Autodesk Inventor part; units mm, degrees
ref_plane "YZ Plane" through (0, 0, 0) normal (1, 0, 0) x (0, 1, 0)
ref_plane "XZ Plane" through (0, 0, 0) normal (0, 1, 0) x (-1, 0, 0)
ref_plane "XY Plane" through (0, 0, 0) normal (0, 0, 1) x (1, 0, 0)
sketch "Sketch1" plane through (0, 0, 0) normal (0, 0, 1) x (1, 0, 0)
  line L0 (0, 0) -> (0, 20)
  line L1 (0, 0) -> (20, 0)
  line L2 (0, 20) -> (3, 20)
  line L3 (3, 20) -> (3, 17)
  line L4 (3, 17) -> (17, 3)
  line L5 (17, 3) -> (20, 3)
  line L6 (20, 3) -> (20, 0)
  dimension "d0" = 20
  dimension "d1" = 20
  dimension "d2" = 3
  dimension "d3" = 3
  dimension "d4" = 3
  dimension "d5" = 3
extrude "Extrusion1" add sketch "Sketch1" along normal mid plane 20
sketch "Sketch2" plane through (0, 20, 10) normal (0, 1, 0) x (1, 0, 0)
  line L0 (3, 2) -> (17, 2)
  line L1 (17, 2) -> (17, 18)
  line L2 (17, 18) -> (3, 18)
  line L3 (3, 18) -> (3, 2)
  line L4 (0, 0) -> (0, 20)
  line L5 (3, 0) -> (3, 20)
  line L6 (17, 0) -> (17, 20)
  line L7 (3, 20) -> (17, 20)
  point P0 (0, 10)
  point P1 (3, 10)
  point P2 (0, 10)
  dimension "d8" = 2
extrude "Extrusion2" cut sketch "Sketch2" against normal up to surface (17 mm away) contours L3 L2 L1 L0
sketch "Sketch3" plane through (17, 3, 10) normal (0, 1, 0) x (1, 0, 0)
  line L0 (-10, 10) -> (-3, 10) construction
  line L1 (-10, 8) -> (-3, 8)
  line L2 (-3, 12) -> (-10, 12)
  arc A0 (-10, 12) -> (-10, 8) centre (-10, 10) ccw
  arc A1 (-3, 8) -> (-3, 12) centre (-3, 10) ccw
  line L3 (-17, 0) -> (-17, 20)
  line L4 (-14, 0) -> (-14, 20)
  line L5 (3, 0) -> (3, 20)
  point P0 (-17, 10)
  point P1 (-6.5, 10)
  point P2 (-17, 10)
  point P3 (-17, 10)
  dimension "d11" = 4
  dimension "d12" = 4
  dimension "d21" = 6
extrude "Extrusion3" cut sketch "Sketch3" against normal through all
sketch "Sketch4" plane through (3, 17, 10) normal (1, 0, 0) x (0, 0, -1)
  line L0 (10, -3) -> (10, -10) construction
  line L1 (8, -3) -> (8, -10)
  line L2 (12, -10) -> (12, -3)
  arc A0 (12, -3) -> (8, -3) centre (10, -3) ccw
  arc A1 (8, -10) -> (12, -10) centre (10, -10) ccw
  line L3 (0, -17) -> (20, -17)
  line L4 (0, -14) -> (20, -14)
  line L5 (0, 3) -> (20, 3)
  point P0 (10, -17)
  point P1 (10, -6.5)
  point P2 (10, -17)
  dimension "d16" = 4
  dimension "d17" = 4
  dimension "d18" = 6
extrude "Extrusion4" cut sketch "Sketch4" against normal through all
equation "\"d1\" = d0"
equation "\"d5\" = d2"
properties part number "GUSSET 2020"
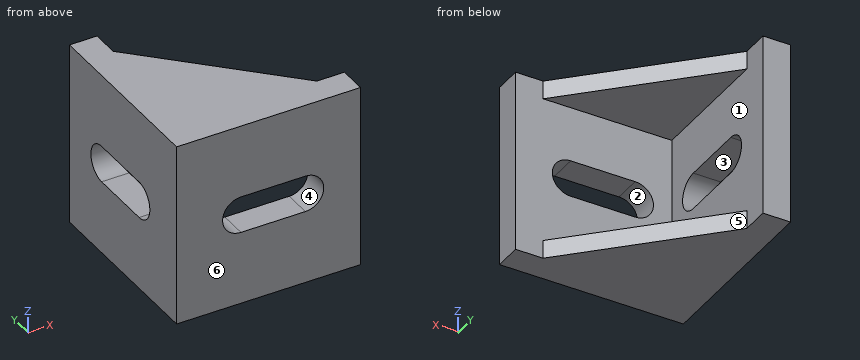
Source: CAD feature listing. Evaluate the final solid. Frame: model axes, mm. Face numbers are marked on the shaded views. A direction names the side the tool comes from. Give positions to 0.01 mm unless a question says otherwise; leave off trailing zeros. Write each loop counter-clockwise with the first axis right and the second up, starting at its lowest first coordinate (ties: lowest second). Pieces come first, ordered by that corner, then holes. Notation, with made-up numbers: (63, -37) - (116, -37) arc R22 ccw to (116, -26) - close; hole circle Ø7 at (33, -21). An arc over 180 degrees is marked (long way). One line per item, written item: value. Start each with the question number.
Q1. Section query B-B, the plane z = 0. Return the cut outline in (x, y).
Q2. Section query A-A, the plane x = 7.5. Return the cut outline in (y, z).
Q3. First-contact query: pin 1 Ø2 at (y, z) = (6.5, 7.5) entering from -X; pin 2 Ø2 at (y, z) = (14.5, 6.5) entering from +X; pin 3 Ø8.5 at (x, z) = (7.5, 0) entering from +Y. Flat tips, straight axial feed; report the tip coordinate or a pass-through.
Q4. Section query C-C, the plane x = 2.25. Return the cut outline in (y, z).
Q5. Draft query along X for the marked faces 4, 5 and 6. Return one class per face: +X half, -X half, draft (parallel to the pull), parting line (faces both ways), or undercut.
Q6. Material intervals for probe 1 along Z at (x, y) = (14.25, 5.5); probe 2 along Y at (x, z) = (5, -5.75); probe 3 along Z at (x, y) = (2, 10.5), sorted ascending. Write a range as from..to.
Q7. Set-up query: the marked faces 1, 2 and 3. Return all of +Z, -Z, +X, -X, +Y, -Y with unobstructed straight access to the full face (end or side cutting, diameter ignored); none if empty.
Q8. Section query D-D, the plane z = 8.75. Return the cut outline in (x, y), then the cut area to 3 significant figures.
Answer:
1. outline: (0, 0) - (5, 0) - (5, 3) - (3, 3) - (3, 5) - (0, 5) - close; (0, 16) - (3, 16) - (3, 20) - (0, 20) - close; (16, 0) - (20, 0) - (20, 3) - (16, 3) - close
2. outline: (0, -10) - (12.5, -10) - (12.5, -8) - (3, -8) - (3, -2) - (0, -2) - close; (0, 2) - (3, 2) - (3, 8) - (12.5, 8) - (12.5, 10) - (0, 10) - close
3. pin 1: stops at x = 0
3. pin 2: stops at x = 3
3. pin 3: stops at y = 3
4. outline: (0, -10) - (20, -10) - (20, 10) - (0, 10) - close; hole (7, -2) - (14, -2) arc R2 ccw to (14, 2) - (7, 2) arc R2 ccw to start
5. face 4: undercut
5. face 5: +X half
5. face 6: draft
6. probe 1: z = -10..-8, 8..10
6. probe 2: y = 0..3
6. probe 3: z = -10..-2, 2..10
7. face 1: +X, +Y
7. face 2: +Y, -Y
7. face 3: +X, -X
8. outline: (0, 0) - (20, 0) - (20, 3) - (17, 3) - (3, 17) - (3, 20) - (0, 20) - close
8. area: 209 mm2
